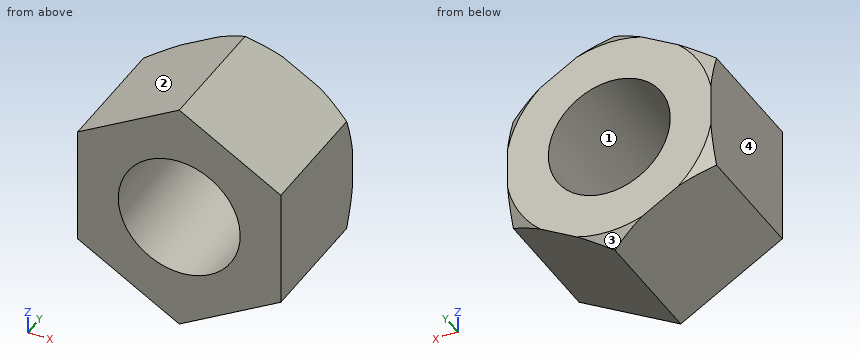
```python
from build123d import *

# Parameters (mm, degrees)
BOSS_EXTRUDE1_DEPTH = 10
SKETCH2_R           = 4.5
CUT_EXTRUDE1_DEPTH  = 10


with BuildPart() as part:
    # Sketch1 → Boss-Extrude1 (new body)
    with BuildSketch(Plane(origin=(0, 0, 0), x_dir=(1, 0, 0), z_dir=(0, 1, 0))):
        Polygon((7.5, 4.330127019), (0, 8.660254038), (-7.5, 4.330127019), (-7.5, -4.330127019), (0, -8.660254038), (7.5, -4.330127019), align=None)
    extrude(amount=BOSS_EXTRUDE1_DEPTH)

    # Sketch3 → Cut-Revolve1 (revolve, cut)
    with BuildSketch(Plane(origin=(0, 0, 0), x_dir=(0, 0, -1), z_dir=(1, 0, 0))):
        Polygon((-8.660254038, 10), (-7.660254038, 10), (-8.660254038, 9.2), align=None)
    revolve(axis=Axis((0, 0, 0), (0, 1, 0)), mode=Mode.SUBTRACT)

    # Sketch2 → Cut-Extrude1 (cut)
    with BuildSketch(Plane(origin=(0, 10, 0), x_dir=(1, 0, 0), z_dir=(0, 1, 0))):
        with Locations(Location((0, 0, 0), (0, 0, 270))):
            Circle(SKETCH2_R)
    extrude(amount=-CUT_EXTRUDE1_DEPTH, mode=Mode.SUBTRACT)


solid = part.part
```
CAD build for the part. Positions are in the model's coordinates, mm. Face numbers are marked on the shaded views. Round coordinates to 2 decimals unless told otherwise and drop trailing zeros. Write each loop counter-clockwise with the first axis right and the second up, starting at its lowest first coordinate (ties: lowest second). Pieces come first, ordered by that corner, then holes. Notation, with made-up numbers: M 48,38.5 L 65,38.5 A20 ccw 65,51.5 Z; hole C -26,55.25 d3. An arc over 180 degrees is marked long. One line per question, with ' | ' between items.
1. Probe L1, parallel to X at y = 2.25, z = 0; L2, parallel to Z at x = -4, y = 4.75; L3, parallel to Z at x = -3.5, y = 3.75. List the from-to ranges inside material, lowest first. Write a range as from..to.
Working result:
L1: -7.5..-4.5, 4.5..7.5 | L2: -6.35..-2.06, 2.06..6.35 | L3: -6.64..-2.83, 2.83..6.64
2. Pin check, flat tips, straight feed: pin 1 Ø6 at (x, y) = (3.5, 9) entering from -Z; pin 2 Ø6 at (x, y) = (0, 3) entering from +Z; pin 3 Ø1 at (x, y) = (-5, 9) entering from -Z. Stop position of each tip, or through.
Working result:
pin 1: z = -8.37 | pin 2: z = 8.66 | pin 3: z = -6.06
3. Cut at C-C on z = 6.25. Write the cut outline in (x, y).
Working result:
outline: M -4.17,0 L 4.17,0 L 4.17,10 L -4.17,10 Z
4. Mould opens along Z. For the marked faces 1, 2, 3 and 4 say: pulls with the +Z half, pulls with the -Z half, needs draft (parallel to the pull), parting line crosses it, or undercut.
Working result:
face 1: undercut | face 2: pulls with the +Z half | face 3: pulls with the -Z half | face 4: needs draft
5. Cut at A-A on y = 5. Write the cut outline in (x, z), and give its area (3 significant figures).
Working result:
outline: M -7.5,-4.33 L 0,-8.66 L 7.5,-4.33 L 7.5,4.33 L 0,8.66 L -7.5,4.33 Z; hole C 0,0 d9 | area: 131 mm2
6. Cut at B-B on z = 0. Write the cut outline in (x, y).
Working result:
outline: M -7.5,0 L -4.5,0 L -4.5,10 L -7.5,10 Z; M 4.5,0 L 7.5,0 L 7.5,10 L 4.5,10 Z
